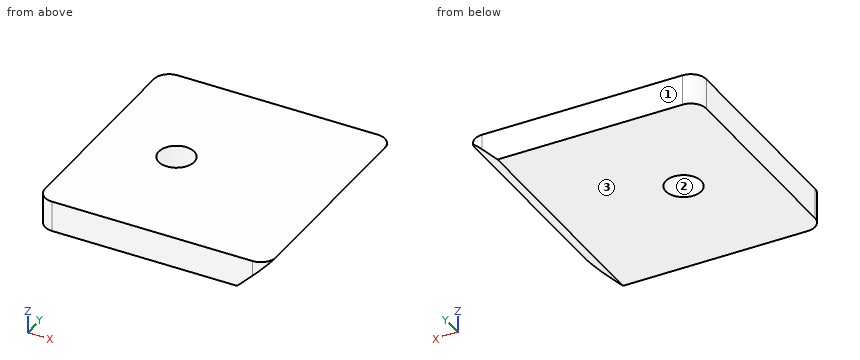
from build123d import *

# Parameters (mm, degrees)
F0_R        = 1.4605
F1_DEPTH    = 2.54
F2_T1_DEPTH = 29.5741495789


# Not quite as in the source:
# - a fillet or chamfer that OpenCascade refuses, or shapes differently, is made with other operations: its cross-section is extruded or revolved along the edge and cut away or added
# - a feature names something its author has since deleted; it is built from what else it names


with BuildPart() as f1:
    # F0 (on Top) → F1 (new body)
    with BuildSketch(Plane.XY):
        with BuildLine():
            Line((-20.32, 2.54), (-3.81, 2.54))
            ThreePointArc((-3.81, 2.54), (-2.9119743879, 2.9119743879), (-2.54, 3.81))
            Line((-2.54, 3.81), (-2.54, 20.32))
            ThreePointArc((-2.54, 20.32), (-2.9119743879, 21.2180256121), (-3.81, 21.59))
            Line((-3.81, 21.59), (-20.32, 21.59))
            ThreePointArc((-20.32, 21.59), (-21.2180256121, 21.2180256121), (-21.59, 20.32))
            Line((-21.59, 20.32), (-21.59, 3.81))
            ThreePointArc((-21.59, 3.81), (-21.2180256121, 2.9119743879), (-20.32, 2.54))
        make_face()
        with Locations((-15.24, 12.065)):
            Circle(F0_R, mode=Mode.SUBTRACT)
    extrude(amount=F1_DEPTH)

    # F2: chamfer of 2.54 on 1 edges, made by hand

    # F2_s2 → F2_t1 (cut)
    with BuildSketch(Plane.XZ.offset(-26.8520747894)):
        Polygon((-2.54, 2.54), (-5.08, 0), (-2.54, 0), align=None)
    extrude(amount=F2_T1_DEPTH, mode=Mode.SUBTRACT)


solid = f1.part
Input: part model. Units: mm. Frame: model coordinates. Face numbers are marked on the shaded views. Coordinates: 2 decimals unless noted, no trailing zeros. Order: outer loops, then holes, each group sorted by start corner. A loop starts at its lowest first (then second) coordinate and runs counter-clockwise, first axis right, second up. Notation, with made-up numbers: M 6,52 L 28,52 A32 ccw 28,90 Z; hole C 21,-10 d5. An arc over 180 degrees is marked long. Answer as CSV lines item,"result".
1. Section A-A (x = -15.24). Return the cut outline in (y, z).
Reported:
outline,"M 2.54,0 L 10.6,0 L 10.6,2.54 L 2.54,2.54 Z; M 13.53,0 L 21.59,0 L 21.59,2.54 L 13.53,2.54 Z"
2. Section C-C (y = 11.25). Return the cut outline in (x, z), then the cut area to 3 significant figures.
Reported:
outline,"M -21.59,0 L -16.45,0 L -16.45,2.54 L -21.59,2.54 Z; M -14.03,0 L -5.08,0 L -2.54,2.54 L -14.03,2.54 Z"
area,"39.0 mm2"
3. Material intervals for line 1 (Y direction, x = -15.24, z = 1.2); line 2 (Y direction, x = -3.75, z = 1.7); line 3 (Y direction, x = -14.5, z = 2.1), sorted ascending. Write a range as from..to.
Reported:
line 1,"2.54..10.6, 13.53..21.59"
line 2,"2.54..21.59"
line 3,"2.54..10.81, 13.32..21.59"
4. Section D-D (x = -4.5). Return the cut outline in (y, z), then the cut area to 3 significant figures.
Reported:
outline,"M 2.54,0.58 L 21.59,0.58 L 21.59,2.54 L 2.54,2.54 Z"
area,"37.3 mm2"
5. Pull-direction query (Y, two-part tool) for the marked faces 1, 2 and 3; classes: released by +Y, released by -Y, zero draft, split by the parting line, or undercut.
Reported:
face 1,"released by +Y"
face 2,"undercut"
face 3,"zero draft"
6. Section B-B (z = 0.25). Return the cut outline in (x, y) (1 decimal).
Reported:
outline,"M -21.6,3.8 A1.3 ccw -20.3,2.5 L -4.8,2.5 L -4.8,21.6 L -20.3,21.6 A1.3 ccw -21.6,20.3 Z; hole C -15.2,12.1 d2.9"
7. First-contact query: P1, Ø1.8, axis at x = -15.24, y = 12.065, coming from the +Z side. Flat tip, straight axial feed; report the tip coordinate or a pass-through.
Reported:
P1,"through"
